Input: part model. Units: mm. Frame: model coordinates. Round coordinates to 2 decimals unless told otherwise and drop trailing zeros. Write each loop counter-clockwise with the first axis right and the second up, starting at its lowest first coordinate (ties: lowest second). Pieces come first, ordered by that corner, then holes. Notation, with made-up numbers: (54, -22.75) -> (58, -22.75) arc R36 cw to (58, 15.25) -> close; hole circle Ø6 at (60.5, 60). An arc over 180 degrees is marked (long way). Write item = value, one per line.
```python
from build123d import *

# Parameters (mm, degrees)
SKETCH3_W            = 120
SKETCH3_H            = 120
BOSS_EXTRUDE2_DEPTH  = 8
SKETCH5_R            = 12.5
CUT_EXTRUDE1_DEPTH   = 9
SKETCH6_R            = 5
CUT_EXTRUDE2_DEPTH   = 9
LPATTERN1_COUNT      = 2
LPATTERN1_PITCH      = 80
LPATTERN1_COUNT_DIR2 = 2
LPATTERN1_PITCH_DIR2 = 80


with BuildPart() as part:
    # Sketch3 → Boss-Extrude2 (new body)
    with BuildSketch(Plane(origin=(0, 0, 0), x_dir=(1, 0, 0), z_dir=(0, 1, 0))):
        Rectangle(SKETCH3_W, SKETCH3_H)
    extrude(amount=BOSS_EXTRUDE2_DEPTH)

    # Sketch5 → Cut-Extrude1 (cut, through all)
    with BuildSketch(Plane(origin=(0, 8, 0), x_dir=(1, 0, 0), z_dir=(0, 1, 0))):
        Circle(SKETCH5_R)
    extrude(amount=-CUT_EXTRUDE1_DEPTH, mode=Mode.SUBTRACT)

    # Sketch6 → Cut-Extrude2 (cut, through all)
    with BuildSketch(Plane(origin=(0, 8, 0), x_dir=(1, 0, 0), z_dir=(0, 1, 0))):
        with Locations((-40, 40)):
            Circle(SKETCH6_R)
    cut_extrude2 = extrude(amount=-CUT_EXTRUDE2_DEPTH, mode=Mode.SUBTRACT)

    # LPattern1: Cut-Extrude2 2 × 2
    with Locations(*[(j * LPATTERN1_PITCH_DIR2, 0, i * LPATTERN1_PITCH) for i in range(LPATTERN1_COUNT) for j in range(LPATTERN1_COUNT_DIR2) if (i, j) != (0, 0)]):
        add(cut_extrude2, mode=Mode.SUBTRACT)


solid = part.part
```
1) Cut plane A-A (x = 40). Return the cut outline in (y, z).
Solutions:
outline = (0, -60) -> (8, -60) -> (8, -45) -> (0, -45) -> close; (0, -35) -> (8, -35) -> (8, 35) -> (0, 35) -> close; (0, 45) -> (8, 45) -> (8, 60) -> (0, 60) -> close
2) Line query: L1, parallel to Z at x = 40, y = 7.25; L2, parallel to Z at x = 0, y = 2.75. Output: solid intervals per line, ascending. Write a range as from..to.
Solutions:
L1 = -60..-45, -35..35, 45..60
L2 = -60..-12.5, 12.5..60
3) Cut plane C-C (z = 7.5). Return the cut outline in (x, y).
Solutions:
outline = (-60, 0) -> (-10, 0) -> (-10, 8) -> (-60, 8) -> close; (10, 0) -> (60, 0) -> (60, 8) -> (10, 8) -> close
4) Cut plane B-B (z = 40). Return the cut outline in (x, y).
Solutions:
outline = (-60, 0) -> (-45, 0) -> (-45, 8) -> (-60, 8) -> close; (-35, 0) -> (35, 0) -> (35, 8) -> (-35, 8) -> close; (45, 0) -> (60, 0) -> (60, 8) -> (45, 8) -> close
5) Cut plane D-D (y = 5.75). Return the cut outline in (x, z).
Solutions:
outline = (-60, -60) -> (60, -60) -> (60, 60) -> (-60, 60) -> close; hole circle Ø10 at (-40, -40); hole circle Ø10 at (-40, 40); hole circle Ø25 at (0, 0); hole circle Ø10 at (40, -40); hole circle Ø10 at (40, 40)
